Model file for the job. Use its own axes, mm. A direction names the side the tool comes from. Round coordinates to 2 decimals unless told otherwise and drop trailing zeros. Order: outer loops, then holes, each group sorted by start corner. A loop starts at its lowest first (then second) coordinate and runs counter-clockwise, first axis right, second up. Notation, with made-up numbers: (73.25, -17.5) -> (100.25, -17.5) arc R19 cw to (100.25, 16.5) -> close; hole circle Ø11 at (15.25, -33). An arc over 180 degrees is marked (long way). Put each result on its own line as item: value. Start each with the question number.
Q1. Flat gauge pins, fed straight in: P1, Ø1, axis at x = 0, y = 1, coming from the +Z side; P2, Ø2, axis at x = -1.5, y = -1.5, coming from the -Z side; P3, Ø1.5, axis at x = -1, y = 1, coming from the +Z side; P4, Ø1, axis at x = 1.5, z = -14.5, coming from the -Y side. Where does each tip first touch, or does it go through?
Q2. Cut at C-C, the plane z = -22. List the corners of the cut face in (x, y), and give its area (3 significant figures).
Q3. Cut at D-D, the plane y = -2.75. List the corners of the cut face in (x, z).
Q4. Cut at A-A, the plane y = 0. List the corners of the cut face in (x, z) (1 decimal).
Q5. Probe L1, parallel to Z at x = 0, y = 2.5; L2, parallel to X at y = -0.5, z = -52; L3, parallel to Y at x = -0.25, z = -30.5. List the from-to ranges inside material, lowest first.
Q6. 3-axis set-ups, long thin cutter, end or side, ignore diameter. For faces 1 (the face through (3.233, -1.341, 0.493)), 2 (the face through (1.5, 0.07, -27.12)): which of +Z, -Z, +X, -X, +Y, -Y reach the whole face in a straight line?
from build123d import *

# Parameters (mm, degrees)
SKETCH1_R           = 3.5
BOSS_EXTRUDE1_DEPTH = 1
DOME1_FACE_RADIUS   = 3.5
DOME1_HEIGHT        = 2
SKETCH3_R           = 1.5
BOSS_EXTRUDE2_DEPTH = 55


with BuildPart() as part:
    # Sketch1 → Boss-Extrude1 (new body)
    with BuildSketch(Plane.XY):
        Circle(SKETCH1_R)
    extrude(amount=BOSS_EXTRUDE1_DEPTH)

    # Dome1: a dome of height H over a round flat face of radius A is a cap of a sphere of radius (A * A + H * H) / (2 * H)
    dome1_r = (DOME1_FACE_RADIUS * DOME1_FACE_RADIUS + DOME1_HEIGHT * DOME1_HEIGHT) / (2 * DOME1_HEIGHT)
    dome1_base = Plane((0, 0, 1), z_dir=(0, 0, 1))
    with Locations(dome1_base.offset(DOME1_HEIGHT - dome1_r)):
        dome1_ball = Sphere(dome1_r, mode=Mode.PRIVATE)
    add(split(dome1_ball, bisect_by=dome1_base, keep=Keep.TOP, mode=Mode.PRIVATE))

    # Sketch3 → Boss-Extrude2 (add)
    with BuildSketch(Plane(origin=(0, 0, 0), x_dir=(-1, 0, 0), z_dir=(0, 0, -1))):
        Circle(SKETCH3_R)
    extrude(amount=BOSS_EXTRUDE2_DEPTH)


solid = part.part
Ans:
1. P1: stops at z = 2.97
1. P2: stops at z = -55
1. P3: stops at z = 2.95
1. P4: stops at y = -1.12
2. outline: circle Ø3 at (0, 0)
2. area: 7.07 mm^2
3. outline: (-2.17, 0) -> (2.17, 0) -> (2.17, 1) arc R2.99 ccw to (-2.17, 1) -> close
4. outline: (-3.5, 0) -> (-1.5, 0) -> (-1.5, -55) -> (1.5, -55) -> (1.5, 0) -> (3.5, 0) -> (3.5, 1) arc R4.1 ccw to (-3.5, 1) -> close
5. L1: z = 0 to 2.14
5. L2: x = -1.41 to 1.41
5. L3: y = -1.48 to 1.48
6. face 1: +Z, -Z
6. face 2: -Z
